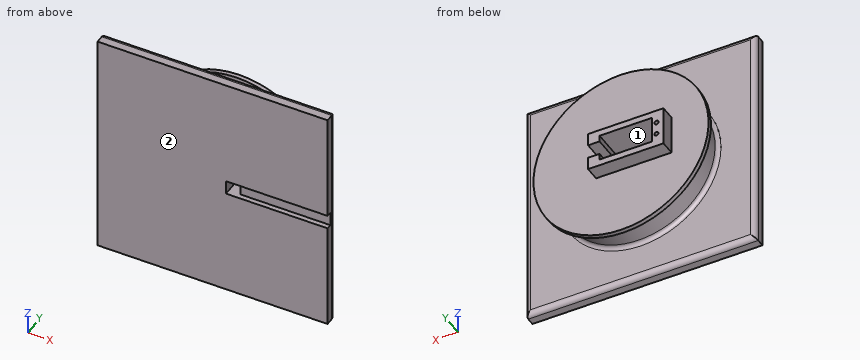
from build123d import *

# Parameters (mm, degrees)
ESQUISSE1_W             = 180
ESQUISSE1_H             = 180
CARR_DEPTH              = 10
ESQUISSE2_R             = 60
ROND_DEPTH              = 28
CONG_2_R                = 4
CONG_8_R                = 3
ESQUISSE27_R            = 68.5
BOSS_EXTRU_2_DEPTH      = 3.5
ESQUISSE20_W            = 41
ESQUISSE20_H            = 21
ENL_V_MAT_EXTRU_1_DEPTH = 15
ESQUISSE21_W            = 59
ESQUISSE21_H            = 31
ESQUISSE21_W_2          = 41
ESQUISSE21_H_2          = 21
BOSS_EXTRU_1_DEPTH      = 26.5
D_GAGEMENT_M31_D        = 3.2
D_GAGEMENT_M31_DEPTH    = 4
D_GAGEMENT_M31_TIP      = 0.96137699
ENL_V_MAT_EXTRU_2_REACH = 138.566
ESQUISSE25_W            = 9
ESQUISSE25_H            = 11
ESQUISSE26_W            = 11
ESQUISSE26_H            = 4
ENL_V_MAT_EXTRU_3_DEPTH = 151.134939305


with BuildPart() as part:
    # Esquisse1 → Carré (new body)
    with BuildSketch(Plane(origin=(0, 0, 0), x_dir=(1, 0, 0), z_dir=(0, 1, 0))):
        Rectangle(ESQUISSE1_W, ESQUISSE1_H)
    extrude(amount=CARR_DEPTH)

    # Esquisse2 → Rond (add)
    with BuildSketch(Plane(origin=(0, 10, 0), x_dir=(1, 0, 0), z_dir=(0, 1, 0))):
        with Locations(Location((0, 0, 0), (0, 0, 270))):
            Circle(ESQUISSE2_R)
    extrude(amount=ROND_DEPTH)

    # Congé2
    cong_2_edges = [part.edges().sort_by_distance(p)[0] for p in [
        (-90, 10, 0),
        (0, 10, 90),
        (90, 10, 0),
        (0, 10, -90),
    ]]
    fillet(cong_2_edges, radius=CONG_2_R)

    # Congé8
    cong_8_edges = [part.edges().sort_by_distance(p)[0] for p in [
        (0, 10, -60),
    ]]
    fillet(cong_8_edges, radius=CONG_8_R)

    # Esquisse27 → Boss.-Extru.2 (add)
    with BuildSketch(Plane(origin=(0, 38, 0), x_dir=(1, 0, 0), z_dir=(0, 1, 0))):
        with Locations(Location((0, 0, 0), (0, 0, 270))):
            Circle(ESQUISSE27_R)
    extrude(amount=-BOSS_EXTRU_2_DEPTH)

    # Esquisse20 → Enlèv. mat.-Extru.1 (cut)
    with BuildSketch(Plane(origin=(0, 38, 0), x_dir=(1, 0, 0), z_dir=(0, 1, 0))):
        with Locations((-10, 0)):
            Rectangle(ESQUISSE20_W, ESQUISSE20_H)
    extrude(amount=-ENL_V_MAT_EXTRU_1_DEPTH, mode=Mode.SUBTRACT)

    # Esquisse21 → Boss.-Extru.1 (add)
    with BuildSketch(Plane(origin=(0, 23, 0), x_dir=(1, 0, 0), z_dir=(0, 1, 0))):
        with Locations((-10, 0)):
            Rectangle(ESQUISSE21_W, ESQUISSE21_H)
        with Locations((-10, 0)):
            Rectangle(ESQUISSE21_W_2, ESQUISSE21_H_2, mode=Mode.SUBTRACT)
    extrude(amount=BOSS_EXTRU_1_DEPTH)

    # Dégagement M31
    with Locations(Plane(origin=(0, 49.5, 0), x_dir=(1, 0, 0), z_dir=(0, 1, 0))):
        with Locations((-34, 4.95), (-34, -4.95)):
            Hole(D_GAGEMENT_M31_D / 2, depth=D_GAGEMENT_M31_DEPTH)
            with Locations((0, 0, -(D_GAGEMENT_M31_DEPTH + D_GAGEMENT_M31_TIP / 2))):  # 118° drill point
                Cone(0, D_GAGEMENT_M31_D / 2, D_GAGEMENT_M31_TIP, mode=Mode.SUBTRACT)

    # Enlèv. mat.-Extru.2: up to this face of the body (flat: up to its plane)
    enl_v_mat_extru_2_end = Plane(part.part.faces().sort_by_distance((0, 0, 0))[0])
    # Esquisse25 → Enlèv. mat.-Extru.2 (cut, up to the picked face)
    with BuildSketch(Plane(origin=(0, 49.5, 0), x_dir=(1, 0, 0), z_dir=(0, 1, 0)), mode=Mode.PRIVATE) as enl_v_mat_extru_2_sk1:
        with Locations((15, 0)):
            Rectangle(ESQUISSE25_W, ESQUISSE25_H)
    enl_v_mat_extru_2_tool1 = split(extrude(enl_v_mat_extru_2_sk1.sketch, amount=-ENL_V_MAT_EXTRU_2_REACH, mode=Mode.PRIVATE), bisect_by=enl_v_mat_extru_2_end, keep=Keep.BOTH, mode=Mode.PRIVATE)
    add(enl_v_mat_extru_2_tool1.solids().sort_by(Axis((15, 49.5, 0), (0, -1, 0)))[0], mode=Mode.SUBTRACT)

    # Esquisse26 → Enlèv. mat.-Extru.3 (cut, through all)
    with BuildSketch(Plane.ZY.offset(-19.5)):
        with Locations((0, 2)):
            Rectangle(ESQUISSE26_W, ESQUISSE26_H)
    extrude(amount=-ENL_V_MAT_EXTRU_3_DEPTH, mode=Mode.SUBTRACT)


solid = part.part
Verification items for the finished model (mm, model axes). Face numbers are marked on the shaded views. Give positions to 0.01 mm unless a question says otherwise; leave off trailing zeros. Write each loop counter-clockwise with the first axis right and the second up, starting at its lowest first coordinate (ties: lowest second). Pieces come first, ordered by that corner, then holes. Notation, with made-up numbers: M -27,-1 L 13,-1 A37 cw 13,37 Z; hole C 32.25,-33 d7. An arc over 180 degrees is marked long. Put each result on its own line as item: value. Start each with the question number.
1. Section check B-B (y = 42). Record the cut outline in (x, z), and give its area (3 significant figures).
2. Section check A-A (z = 0). Record the cut outline in (x, y), and give its area (3 significant figures).
3. Section check C-C (x = 0). Record the cut outline in (y, z).
4. Scan lines: line 1 along Z through (x, y) = (-34, 46.95); line 2 along X through (y, z) = (47.9, -4.95); line 3 along Y through (x, z) = (7, 63.5). Record each from-to range of solid material in increasing order. Write a range as [from, to].
5. Section check D-D (y = 31). Record the cut outline in (x, z).
6. Draft check along X on the marked faces 1 and 2. Enter one of: +X half, -X half, draft (parallel to the pull), parting line (faces both ways), or undercut.
7. Go/stop test with flat-tipped pins: pin 1 Ø12.5 at (y, z) = (43.5, 6.5) entering from -X; pin 2 Ø1 at (x, y) = (62, 26) entering from -Z; pin 3 Ø12 at (y, z) = (14.5, -35.5) entering from -X; pin 4 Ø12 at (x, z) = (-56.5, 17.5) entering from +Y. Record where each tip stops, or that it passes through.
Answer list:
1. outline: M -39.5,-15.5 L 19.5,-15.5 L 19.5,-5.5 L 10.5,-5.5 L 10.5,-10.5 L -30.5,-10.5 L -30.5,10.5 L 10.5,10.5 L 10.5,5.5 L 19.5,5.5 L 19.5,15.5 L -39.5,15.5 Z
1. area: 869 mm2
2. outline: M -90,0 L 10.5,0 L 10.5,23 L -30.5,23 L -30.5,49.5 L -39.5,49.5 L -39.5,38 L -68.5,38 L -68.5,34.5 L -60,34.5 L -60,13 A3 cw -63,10 L -86,10 A4 ccw -90,6 Z; M 19.5,4 L 90,4 L 90,6 A4 ccw 86,10 L 63,10 A3 cw 60,13 L 60,34.5 L 68.5,34.5 L 68.5,38 L 19.5,38 Z
2. area: 4,080 mm2
3. outline: M 0,-90 L 6,-90 A4 ccw 10,-86 L 10,-63 A3 cw 13,-60 L 34.5,-60 L 34.5,-68.5 L 38,-68.5 L 38,-15.5 L 49.5,-15.5 L 49.5,-10.5 L 23,-10.5 L 23,10.5 L 49.5,10.5 L 49.5,15.5 L 38,15.5 L 38,68.5 L 34.5,68.5 L 34.5,60 L 13,60 A3 cw 10,63 L 10,86 A4 ccw 6,90 L 0,90 Z
4. line 1: [-15.5, -6.55], [-3.35, 3.35], [6.55, 15.5]
4. line 2: [-39.5, -35.6], [-32.4, -30.5]
4. line 3: [0, 10], [34.5, 38]
5. outline: C 0,0 d120; hole M -30.5,-10.5 L 10.5,-10.5 L 10.5,-5.5 L 19.5,-5.5 L 19.5,5.5 L 10.5,5.5 L 10.5,10.5 L -30.5,10.5 Z
6. face 1: undercut
6. face 2: draft
7. pin 1: x = -68.41
7. pin 2: through
7. pin 3: x = -89.12
7. pin 4: y = 38
